```python
from build123d import *

# Parameters (mm, degrees)
SKETCH1_W               = 480
SKETCH1_H               = 480
BOSS_EXTRUDE1_DEPTH     = 240
FILLET1_R               = 20
SHELL1_T                = -10
SKETCH3_R               = 30
CUT_EXTRUDE1_DEPTH      = 741.337760755
CUT_EXTRUDE1_DEPTH_BACK = 741.337760755
SCALE1_SCALE            = 0.5


with BuildPart() as part:
    # Sketch1 → Boss-Extrude1 (new, symmetric)
    with BuildSketch(Plane.XY):
        with Locations((240, -240)):
            Rectangle(SKETCH1_W, SKETCH1_H)
    extrude(amount=BOSS_EXTRUDE1_DEPTH, both=True)

    # Fillet1
    fillet1_edges = [part.edges().sort_by_distance(p)[0] for p in [
        (480, -240, 240),
        (240, 0, 240),
        (0, -240, 240),
        (240, 0, -240),
        (480, -240, -240),
        (240, -480, -240),
        (0, -240, -240),
        (0, 0, 0),
        (480, 0, 0),
        (480, -480, 0),
        (0, -480, 0),
        (240, -480, 240),
    ]]
    fillet(fillet1_edges, radius=FILLET1_R)

    # Sketch2 → Revolve1 (revolve)
    with BuildSketch(Plane.XY, mode=Mode.PRIVATE) as revolve1_sk:
        Polygon((240, 0), (360, 0), (353, 30), (240, 30), align=None)
        Polygon((360, -480), (353, -510), (240, -510), (240, -480), align=None)
    revolve(revolve1_sk.sketch.rotate(Axis((240, 0, 0), (0, 1, 0)), 90), axis=Axis((240, 0, 0), (0, 1, 0)))

    # Shell1
    shell1_openings = [part.faces().sort_by_distance(p)[0] for p in [
        (240, 30, 0),
        (240, -510, 0),
    ]]
    offset(amount=SHELL1_T, openings=shell1_openings, kind=Kind.INTERSECTION)

    # Sketch3 → Cut-Extrude1 (cut, two sides)
    with BuildSketch(Plane.XY) as cut_extrude1_sk:
        with Locations((240, -55)):
            Circle(SKETCH3_R)
    extrude(amount=CUT_EXTRUDE1_DEPTH, mode=Mode.SUBTRACT)
    extrude(cut_extrude1_sk.sketch, amount=-CUT_EXTRUDE1_DEPTH_BACK, mode=Mode.SUBTRACT)


with BuildPart() as part_1:
    # Scale1: scaled about (0, 0, 0)
    add(part.part.scale(SCALE1_SCALE))


solid = part_1.part
```
For this review, take the finished solid that the model builds, in its own axes (mm). A direction names the side the tool comes from. Round coordinates to 2 decimals unless told otherwise and drop trailing zeros. Write each loop counter-clockwise with the first axis right and the second up, starting at its lowest first coordinate (ties: lowest second). Pieces come first, ordered by that corner, then holes. Notation, with made-up numbers: (26.5, 6.25) - (33.5, 6.25) arc R4 ccw to (33.5, 12.25) - close; hole circle Ø5 at (-35.75, 65.25). An arc over 180 degrees is marked (long way). Put each result on its own line as item: value.
Q1. Machinability: for faces 1 (the face through (70, 0, -47)), 2 (the face through (118, -118, -115)), 3 (the face through (118, -118, 120)), which of the approach directions +Z, -Z, +X, -X, +Y, -Y give a long, thin tool a straight path to every point of the face, cutting with its end or side? Answer none if there is none.
Solved:
face 1: +Y
face 2: none
face 3: +Z, +X, -X, +Y, -Y
Q2. Wall thickness on probe 1 along Y at (x, z) = (209, 30.5); probe 2 along Z at (x, y) = (166.5, -230); probe 3 along X at (y, z) = (-104.5, 80.5): over which ranges is each line inside the solid? List them lowest first.
Solved:
probe 1: y = -240 to -235, -5 to 0
probe 2: z = -120 to -115, 115 to 120
probe 3: x = 0 to 5, 235 to 240
Q3. Mouldability with a two-part tool opening along Z and no side actions: class faces 4 (the face through (5, -122, 2)), 5 (the face through (235, -122, 2)), 6 (the face through (63.812, 14.272, 7.377)), 7 (the face through (121.54, -236.99, 117.15)) as released by +Z, released by -Z, zero draft, split by the parting line, or undercut.
Solved:
face 4: undercut
face 5: undercut
face 6: split by the parting line
face 7: released by +Z
Q4. We need section A-A (y = -27.5). Give the boundary of the cut face in (x, z), and give its area (3 significant figures).
Solved:
outline: (0, -110) arc R10 ccw to (10, -120) - (105, -120) - (105, -115) - (10, -115) arc R5 cw to (5, -110) - (5, 110) arc R5 cw to (10, 115) - (105, 115) - (105, 120) - (10, 120) arc R10 ccw to (0, 110) - close; (135, -120) - (230, -120) arc R10 ccw to (240, -110) - (240, 110) arc R10 ccw to (230, 120) - (135, 120) - (135, 115) - (230, 115) arc R5 cw to (235, 110) - (235, -110) arc R5 cw to (230, -115) - (135, -115) - close
area: 4,340 mm2
Q5. We need section B-B (x = 54). Give the boundary of the cut face in (y, z).
Solved:
outline: (-240, -110) arc R10 ccw to (-230, -120) - (-10, -120) arc R10 ccw to (0, -110) - (0, 110) arc R10 ccw to (-10, 120) - (-230, 120) arc R10 ccw to (-240, 110) - close; hole (-235, -110) arc R5 ccw to (-230, -115) - (-10, -115) arc R5 ccw to (-5, -110) - (-5, 110) arc R5 ccw to (-10, 115) - (-230, 115) arc R5 ccw to (-235, 110) - close
Q6. Insertion check: pin 1 Ø6 at (x, z) = (53.5, 29.5) entering from -Y; pin 2 Ø5 at (x, z) = (36, 53.5) entering from +Y. Each pin has a flat end and moves straight along its axis. Give the tip position at first contact, or say it passes through.
Solved:
pin 1: stops at y = -240
pin 2: stops at y = 0
Q7. We need section C-C (z = 93). Give the boundary of the cut face in (x, y), and give its area (3 significant figures).
Solved:
outline: (0, -230) arc R10 ccw to (10, -240) - (230, -240) arc R10 ccw to (240, -230) - (240, -10) arc R10 ccw to (230, 0) - (10, 0) arc R10 ccw to (0, -10) - close; hole (5, -230) arc R5 ccw to (10, -235) - (230, -235) arc R5 ccw to (235, -230) - (235, -10) arc R5 ccw to (230, -5) - (10, -5) arc R5 ccw to (5, -10) - close
area: 4,640 mm2
